Read the model definition and answer for the solid it produces. Units are mm, in the model's axes. A direction names the side the tool comes from. Round coordinates to 2 decimals unless told otherwise and drop trailing zeros. Order: outer loops, then holes, each group sorted by start corner. A loop starts at its lowest first (then second) coordinate and runs counter-clockwise, first axis right, second up. Notation, with made-up numbers: (71.25, 82.5) -> (77.25, 82.5) arc R29 cw to (77.25, 111.5) -> close; hole circle Ø11 at (39, 72). An arc over 180 degrees is marked (long way). Use a Markdown table: item, result. Add a question column.
1. Consider L1, parallel to X at y = -5.5, z = -1.5; L2, parallel to Z at x = 4.75, y = 0; L3, parallel to Z at x = 0.55, y = -2.75. Determine where each line is inside the solid, lowest interval first. Write a range as [from, to].
2. Given pin 1 (2 mm diameter, centred on x = 2, y = 4.5, fed in from -Z); pin 2 (1.5 mm diameter, centred on x = 3.5, y = -3.5, fed in from -Z); pin 3 (1 mm diameter, centred on x = 1.5, z = -1.5, fed in from +Y), each flat-ended and moving along its own axis, determine where each tip first touches the part or whether it passes through.
3. For faces 4 (the face through (5.55, 0, -6)), 5 (the face through (0, -3, 2)), determine the directions among +Z, -Z, +X, -X, +Y, -Y from which every point of the face is accessible in a straight line to the end or side of a thin tool.
4. Section B-B, the plane x = 3.65 is taken. Give the vertices of the cut face in (y, z), then the cut area to 3 significant figures.
5. The mould has two halves that part along Z. Classify faces 1 (the face through (6, -3, 2)), 2 (the face through (3.04, -0.65, -2.93)), 3 (the face through (4.9, -1, 4.4)): +Z half, -Z half, draft (parallel to the pull), parting line (faces both ways), or undercut.
6. Section A-A, the plane x = 2.85 is taken. Give the vertices of the cut face in (y, z).
Autodesk Inventor part; units mm, degrees
ref_plane "YZ Plane" through (0, 0, 0) normal (1, 0, 0) x (0, 1, 0)
ref_plane "XZ Plane" through (0, 0, 0) normal (0, 1, 0) x (-1, 0, 0)
ref_plane "XY Plane" through (0, 0, 0) normal (0, 0, 1) x (1, 0, 0)
sketch "Sketch_18" plane through (0, 0, 0) normal (0, 0, 1) x (1, 0, 0)
  line L0 (50, 0) -> (-50, 0)
  arc A0 (0, 3.3005) -> (0.3, 3.0005) centre (0.3, 3.3005) ccw
  line L1 (0.3, 3.0005) -> (5.7, 3.0005)
  arc A1 (5.7, 3.0005) -> (6, 3.3005) centre (5.7, 3.3005) ccw
  line L2 (6, 3.3005) -> (6, 4.513)
  line L3 (6, 4.513) -> (4.3303, 4.513)
  arc A2 (1.6697, 4.513) -> (4.3303, 4.513) centre (3, 5.65) ccw
  line L4 (1.6697, 4.513) -> (0, 4.513)
  line L5 (0, 4.513) -> (0, 3.3005)
revolve "Revolution1" add sketch "Sketch_18" angle 360 about axis through (50, 0, 0) along (1, 0, 0)
sketch "Sketch_19" plane through (0, 0, 0) normal (0, 0, 1) x (1, 0, 0)
  line L0 (50, 0) -> (-50, 0)
  line L1 (0, 5.5125) -> (0, 4.1)
  line L2 (0, 4.1) -> (0.2917, 4.1)
  arc A0 (0.2917, 4.1) -> (0.5, 4.3083) centre (0.2917, 4.3083) ccw
  line L3 (0.5, 4.3083) -> (0.5, 5.1792)
  line L4 (0.5, 5.1792) -> (5.5, 5.1792)
  line L5 (5.5, 5.1792) -> (5.5, 4.3083)
  arc A1 (5.5, 4.3083) -> (5.7083, 4.1) centre (5.7083, 4.3083) ccw
  line L6 (5.7083, 4.1) -> (6, 4.1)
  line L7 (6, 4.1) -> (6, 5.5125)
  line L8 (6, 5.5125) -> (0, 5.5125)
revolve "Revolution2" cut sketch "Sketch_19" angle 360 about axis through (50, 0, 0) along (1, 0, 0)
sketch "Sketch_20" plane through (0, 0, 0) normal (0, 0, 1) x (1, 0, 0)
  line L0 (50, 0) -> (-50, 0)
  line L1 (0.27, 7.4) -> (0.315, 6.5725)
  line L2 (0.315, 6.5725) -> (0.27, 5.745)
  line L3 (0.27, 5.745) -> (0.27, 4.09)
  line L4 (0.27, 4.09) -> (0.36, 4.09)
  line L5 (0.36, 4.09) -> (0.45, 5.745)
  line L6 (0.45, 5.745) -> (0.45, 6.5725)
  line L7 (0.45, 6.5725) -> (0.36, 7.4)
  line L8 (0.36, 7.4) -> (0.27, 7.4)
revolve "Revolution3" add sketch "Sketch_20" angle 360 about axis through (50, 0, 0) along (1, 0, 0)
sketch "Sketch_21" plane through (0, 0, 0) normal (0, 0, 1) x (1, 0, 0)
  line L0 (50, 0) -> (-50, 0)
  line L1 (5.55, 6.5725) -> (5.55, 5.745)
  line L2 (5.55, 5.745) -> (5.64, 4.09)
  line L3 (5.64, 4.09) -> (5.73, 4.09)
  line L4 (5.73, 4.09) -> (5.73, 5.745)
  line L5 (5.73, 5.745) -> (5.685, 6.5725)
  line L6 (5.685, 6.5725) -> (5.73, 7.4)
  line L7 (5.73, 7.4) -> (5.64, 7.4)
  line L8 (5.64, 7.4) -> (5.55, 6.5725)
revolve "Revolution4" add sketch "Sketch_21" angle 360 about axis through (50, 0, 0) along (1, 0, 0)
properties part number "W 606-2Z_PART1" material "Stainless Steel"
Verdict:
| question | item | result |
|---|---|---|
| 1 | L1 | x = [0.27, 0.45], [5.55, 5.73] |
| 1 | L2 | z = [-4.51, -3], [3, 4.51] |
| 1 | L3 | z = [-3.58, -1.2], [1.2, 3.58] |
| 2 | pin 1 | stops at z = -2.78 |
| 2 | pin 2 | stops at z = -3.02 |
| 2 | pin 3 | stops at y = 4.4 |
| 3 | face 4 | none |
| 3 | face 5 | +Z, -Z, -X, +Y, -Y |
| 4 | outline | circle Ø8.05 at (0, 0); hole circle Ø6 at (0, 0) |
| 4 | area | 22.6 mm2 |
| 5 | face 1 | draft |
| 5 | face 2 | undercut |
| 5 | face 3 | parting line |
| 6 | outline | circle Ø7.81 at (0, 0); hole circle Ø6 at (0, 0) |
